Print and shaded views of the part. All mm, measured from the part's lowest x, y and z. A direction names the side the tool comes from. Round coordinates to 2 decimals unless told otherwise and drop trailing zeros. Write each loop counter-clockwise with the first axis right and the second up, starting at its lowest first coordinate (ties: lowest second). Pieces come first, ordered by that corner, then holes. Notation, with made-up numbers: (33, 10.5) - (38, 10.5) arc R21 ccw to (38, 15.5) - close; hole circle Ø8 at (22.5, -2.5). An arc over 180 degrees is marked (long way). One line per item, written item: value.
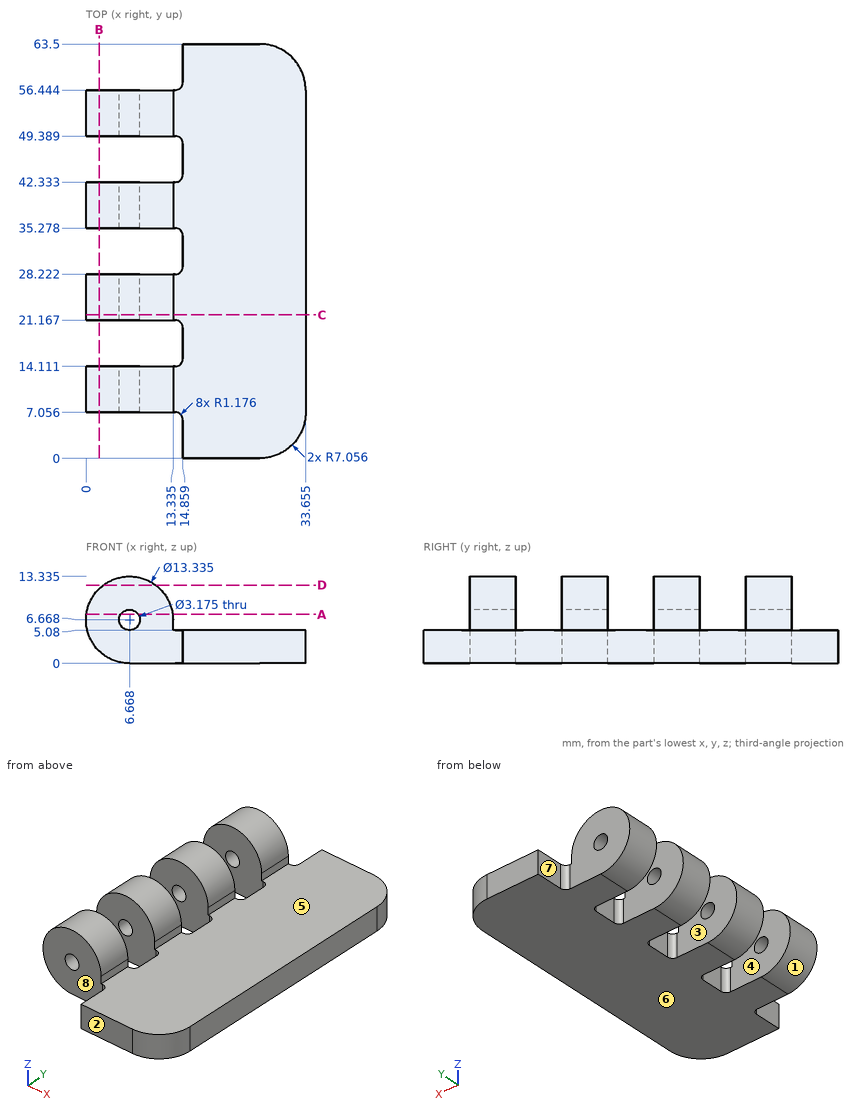
1. Band-saw the part on C-C on y = 22. Write the cut outline in (x, z) (1 decimal).
Report:
outline: (6.7, 0) - (33.7, 0) - (33.7, 5.1) - (13.3, 5.1) - (13.3, 6.7) arc R6.7 ccw (long way) to start; hole circle Ø3.2 at (6.7, 6.7)
2. Band-saw the part on D-D on z = 12. Write the cut outline in (x, y) (1 decimal).
Report:
outline: (2.7, 7.1) - (10.7, 7.1) - (10.7, 14.1) - (2.7, 14.1) - close; (2.7, 21.2) - (10.7, 21.2) - (10.7, 28.2) - (2.7, 28.2) - close; (2.7, 35.3) - (10.7, 35.3) - (10.7, 42.3) - (2.7, 42.3) - close; (2.7, 49.4) - (10.7, 49.4) - (10.7, 56.4) - (2.7, 56.4) - close
3. Tool access for the marked faces 4, 5, 6, 7 and 8: list every direction of +Z, -Z, +X, -X, +Y, -Y with a clear straight run to the whole face (end or side of a thin tool).
Report:
face 4: +Z, -Z, -X
face 5: +Z, +X, +Y, -Y
face 6: -Z, +X, -X, +Y, -Y
face 7: +Z, -Z, -X, +Y
face 8: +Z, -Z, -X, -Y
4. Wall check: probe 1 along Y at (x, z) = (3, 2.5) (1 decimal); probe 2 along Z at (x, y) = (20, 49.5); probe 3 along Z at (x, y) = (7, 51) (1 decimal). Give the ranges that are in metal, low to high. Write a range as [from, to].
Report:
probe 1: [7.1, 14.1], [21.2, 28.2], [35.3, 42.3], [49.4, 56.4]
probe 2: [0, 5.08]
probe 3: [0, 5.1], [8.2, 13.3]
5. Band-saw the part on B-B on x = 2. Write the cut outline in (y, z) (1 decimal), plus the area to 3 significant figures.
Report:
outline: (7.1, 1.9) - (14.1, 1.9) - (14.1, 11.4) - (7.1, 11.4) - close; (21.2, 1.9) - (28.2, 1.9) - (28.2, 11.4) - (21.2, 11.4) - close; (35.3, 1.9) - (42.3, 1.9) - (42.3, 11.4) - (35.3, 11.4) - close; (49.4, 1.9) - (56.4, 1.9) - (56.4, 11.4) - (49.4, 11.4) - close
area: 269 mm²
6. Band-saw the part on A-A on z = 7.5. State how many separate pieces and enclosed holes the cut face has, plus the area to 3 significant figures.
Report:
separate pieces: 8
enclosed holes: 0
area: 297 mm²
7. Mould opens along Y. For the marked faces 1, 2 and 3 say: released by +Y, released by -Y, zero draft, split by the parting line, or undercut.
Report:
face 1: zero draft
face 2: released by -Y
face 3: undercut
8. Drop flat-ended pins along their axis: pin 1 (8 mm diameter, centred on x = 14.5, z = 9.5, fed in from +Y); pin 2 (4 mm diameter, centred on x = 8.5, z = 6, fed in from -Y); pin 3 (3 mm diameter, centred on x = 6.67, z = 6.67, fed in from -Y); pin 4 (1.3 mm diameter, centred on y = 39, z = 6, fed in from +X) (1 decimal). Give the stop position or say it passes through.
Report:
pin 1: y = 56.44
pin 2: y = 7.06
pin 3: through
pin 4: x = 13.3
